Geometry check sheet. Reference: the model listing, model coordinates, mm. Give positions to 0.01 mm unless a question says otherwise; leave off trailing zeros. Loops run counter-clockwise (first coordinate to the right, second up) from the corner with the lowest first, then second, coordinate; pieces in that order, holes last. Notation, with made-up numbers: (12, -7.75) -> (32, -7.75) arc R21 cw to (32, 28.25) -> close; hole circle Ø2 at (43, 16.25). An arc over 180 degrees is marked (long way). Write each question's results on one line, items separated by ' | '. Start each with the question number.
1) Sectioned sample at B-B on x = 0. Record the cut outline in (y, z), then the cut area to 3 significant figures.
2) Sectioned sample at C-C on y = -0.1. Record the cut outline in (x, z), then the cut area to 3 significant figures.
3) Sectioned sample at A-A on z = 0. Record the cut outline in (x, y), then the cut area to 3 significant figures.
4) Depth check by flat-ended pin: pin 1 (1 mm diameter, centred on x = 9.5, y = -0.5, fed in from +Z); pin 2 (1 mm diameter, centred on y = 0, z = -2, fed in from +X). Enter the tip coordinate at first touch or a pass-through.
5) Scan lines: line 1 (Z direction, x = 0, y = -0.4); line 2 (X direction, y = -0.6, z = 1); line 3 (X direction, y = -0.75, z = -2). Record each from-to range of solid material in increasing order. Write a range as from..to.
6) Draft check along Z on faces 1 (the face through (-6, 1, 0)), 2 (the face through (-12.698, 0.014, -4.124)), 3 (the face through (-3.746, -0.014, -0.165)), 4 (the face through (16, 0, 0)). Enter one of: pulls with the +Z half, pulls with the -Z half, needs draft (parallel to the pull), parting line crosses it, or undercut.
7) Sectioned sample at D-D on x = -15.5. Record the cut outline in (y, z), then the cut area to 3 significant figures.
```python
from build123d import *

# Parameters (mm, degrees)
SKETCH1_R           = 3.75
BOSS_EXTRUDE1_DEPTH = 1


with BuildPart() as part:
    # Sketch1 → Boss-Extrude1 (new body, symmetric)
    with BuildSketch(Plane(origin=(0, 0, 0), x_dir=(1, 0, 0), z_dir=(0, 1, 0))):
        with BuildLine():
            Line((-25.27, -2.987825296), (-0.4725, -5.228694268))
            ThreePointArc((-0.4725, -5.228694268), (0.219991794, -5.245388795), (0.908653846, -5.170768626))
            Line((0.908653846, -5.170768626), (13.519230769, -2.954724929))
            ThreePointArc((13.519230769, -2.954724929), (16, 0), (13.519230769, 2.954724929))
            Line((13.519230769, 2.954724929), (0.908653846, 5.170768626))
            ThreePointArc((0.908653846, 5.170768626), (0.219991794, 5.245388795), (-0.4725, 5.228694268))
            Line((-0.4725, 5.228694268), (-25.27, 2.987825296))
            ThreePointArc((-25.27, 2.987825296), (-28, 0), (-25.27, -2.987825296))
        make_face()
        Circle(SKETCH1_R, mode=Mode.SUBTRACT)
    extrude(amount=BOSS_EXTRUDE1_DEPTH, both=True)


solid = part.part
```
Result:
1) outline: (-1, -5.25) -> (1, -5.25) -> (1, -3.75) -> (-1, -3.75) -> close; (-1, 3.75) -> (1, 3.75) -> (1, 5.25) -> (-1, 5.25) -> close | area: 6.00 mm^2
2) outline: (-25.27, -2.99) -> (-0.47, -5.23) arc R5.25 ccw to (0.91, -5.17) -> (13.52, -2.95) arc R3 ccw to (13.52, 2.95) -> (0.91, 5.17) arc R5.25 ccw to (-0.47, 5.23) -> (-25.27, 2.99) arc R3 ccw to start; hole circle Ø7.5 at (0, 0) | area: 300 mm^2
3) outline: (-28, -1) -> (-3.75, -1) -> (-3.75, 1) -> (-28, 1) -> close; (3.75, -1) -> (16, -1) -> (16, 1) -> (3.75, 1) -> close | area: 73.0 mm^2
4) pin 1: z = 3.75 | pin 2: x = 15.6
5) line 1: -5.25..-3.75, 3.75..5.25 | line 2: -27.83..-3.61, 3.61..15.83 | line 3: -27.24..-3.17, 3.17..15.24
6) face 1: needs draft | face 2: pulls with the -Z half | face 3: undercut | face 4: parting line crosses it
7) outline: (-1, -3.87) -> (1, -3.87) -> (1, 3.87) -> (-1, 3.87) -> close | area: 15.5 mm^2
